Model file for the job. Use its own axes, mm. A direction names the side the tool comes from. Give positions to 0.01 mm unless a question says otherwise; leave off trailing zeros. Write each loop counter-clockwise with the first axis right and the second up, starting at its lowest first coordinate (ties: lowest second). Pieces come first, ordered by that corner, then holes. Notation, with made-up numbers: (15.5, 71.25) - (54.5, 71.25) arc R28 ccw to (54.5, 99.25) - close; hole circle Ø5 at (83.5, -12). An arc over 180 degrees is marked (long way). One line per item, written item: value. Start each with the question number.
(1) Drop flat-ended pins along their axis: P1, Ø1, axis at x = -4, z = 0, coming from the -Y side; P2, Ø4, axis at x = 0.5, y = 5.5, coming from the -Z side; P3, Ø0.9, axis at y = -1.5, z = -6.5, coming from the +X side; P4, Ø3, axis at x = 1.5, y = -1, coming from the +Z side. Give the stop position or say it passes through.
(2) Cut at A-A, the plane x = -4.75. List the corners of the cut face in (y, z), and give its area (3 significant figures).
(3) Cut at B-B, the plane y = 2.5. List the corners of the cut face in (x, z).
(4) Cut at D-D, the plane x = 0. List the corners of the cut face in (y, z).
(5) 3-axis set-ups, long thin cutter, end or side, ignore diameter. For faces 1 (the face through (-2.3, 3.1, -3.4)), 2 (the face through (-5.5, 1.5, -5.5)): which of +Z, -Z, +X, -X, +Y, -Y reach the whole face in a straight line?
(6) Cut at C-C, the plane z = 4. List the corners of the cut face in (x, y), and give its area (3 significant figures).
(7) Probe L1, parallel to Y at x = -2, z = 4.75; L2, parallel to Y at x = -5.5, z = 0.75; L3, parallel to Z at x = -2, y = 5. List the from-to ranges inside material, lowest first.
from build123d import *

# Parameters (mm, degrees)
SKETCH1_W            = 12
SKETCH1_H            = 12
BOSS_EXTRUDE1_DEPTH  = 3
CHAMFER1_SIZE        = 1
SKETCH2_W            = 10
SKETCH2_H            = 10
BOSS_EXTRUDE2_DEPTH  = 0.1
SKETCH3_R            = 0.5
BOSS_EXTRUDE3_DEPTH  = 0.05
LPATTERN1_COUNT      = 2
LPATTERN1_PITCH      = 8
LPATTERN1_COUNT_DIR2 = 2
LPATTERN1_PITCH_DIR2 = 8
SKETCH4_R            = 3.5
BOSS_EXTRUDE4_DEPTH  = 8
BOSS_EXTRUDE4_TAPER  = 4
SWEEP1_START         = -3
SWEEP1_DEPTH         = 1
SWEEP1_START_2       = 2
SWEEP1_2_DEPTH       = 1


# Read off the part's stored shape, not the designer's step: Dome1, Sweep1
with BuildPart() as part:
    # Sketch1 → Boss-Extrude1 (new body)
    with BuildSketch(Plane(origin=(0, 0, 0), x_dir=(1, 0, 0), z_dir=(0, 1, 0))):
        Rectangle(SKETCH1_W, SKETCH1_H)
    extrude(amount=BOSS_EXTRUDE1_DEPTH)

    # Chamfer1
    chamfer1_edges = [part.edges().sort_by_distance(p)[0] for p in [
        (6, 1.5, 6),
        (-6, 1.5, 6),
        (-6, 1.5, -6),
        (6, 1.5, -6),
    ]]
    chamfer(chamfer1_edges, length=CHAMFER1_SIZE)

    # Sketch2 → Boss-Extrude2 (add)
    with BuildSketch(Plane(origin=(0, 3, 0), x_dir=(1, 0, 0), z_dir=(0, 1, 0))):
        Rectangle(SKETCH2_W, SKETCH2_H)
    extrude(amount=BOSS_EXTRUDE2_DEPTH)

    # Sketch3 → Boss-Extrude3 (add)
    with BuildSketch(Plane(origin=(0, 3.1, 0), x_dir=(1, 0, 0), z_dir=(0, 1, 0))):
        with Locations(Location((-4, 4, 0), (0, 0, 270))):
            Circle(SKETCH3_R)
    boss_extrude3 = extrude(amount=BOSS_EXTRUDE3_DEPTH)

    # Dome1 outline → Dome1 (revolve)
    with BuildSketch(Plane(origin=(-4, 0, -4), x_dir=(1, 0, 0), z_dir=(0, 0, 1))):
        with BuildLine():
            Line((0, 3.15), (0.5, 3.149999999))
            ThreePointArc((0.5, 3.149999999), (0.353553391, 3.50355339), (0, 3.65))
            Line((0, 3.65), (0, 3.15))
        make_face()
    dome1 = revolve(axis=Axis((-4, 0, -4), (0, 1, 0)))

    # LPattern1: Boss-Extrude3, Dome1 2 × 2
    with Locations(*[(i * LPATTERN1_PITCH, 0, j * LPATTERN1_PITCH_DIR2) for i in range(LPATTERN1_COUNT) for j in range(LPATTERN1_COUNT_DIR2) if (i, j) != (0, 0)]):
        add(boss_extrude3)
        add(dome1)

    # Sketch4 → Boss-Extrude4 (add)
    with BuildSketch(Plane(origin=(0, 3.1, 0), x_dir=(1, 0, 0), z_dir=(0, 1, 0))):
        Circle(SKETCH4_R)
    extrude(amount=BOSS_EXTRUDE4_DEPTH, taper=BOSS_EXTRUDE4_TAPER)

    # Sweep1 outline → Sweep1 (add)
    with BuildSketch(Plane.YZ.offset(SWEEP1_START)):
        Polygon((0.75, 6), (-2.007966225, 6.818182656), (-4.321335721, 6.310463619), (-4.306093498, 6.241014001), (-2.010621634, 6.744805015), (0.5, 6), align=None)
    sweep1 = extrude(amount=SWEEP1_DEPTH)

    # Sweep1 2 outline → Sweep1 2 (add)
    with BuildSketch(Plane.YZ.offset(SWEEP1_START_2)):
        Polygon((0.75, 6), (-2.007966225, 6.818182656), (-4.321335721, 6.310463619), (-4.306093498, 6.241014001), (-2.010621634, 6.744805015), (0.5, 6), align=None)
    sweep1_2 = extrude(amount=SWEEP1_2_DEPTH)

    # Mirror1: Sweep1, Sweep1 2 across plane
    add(sweep1.mirror(Plane.XY))
    add(sweep1_2.mirror(Plane.XY))


solid = part.part
Answers follow:
1. P1: stops at y = 0
1. P2: stops at z = -3.47
1. P3: stops at x = 3
1. P4: stops at z = 6.82
2. outline: (0, -6) - (3, -6) - (3, -5) - (3.1, -5) - (3.1, 5) - (3, 5) - (3, 6) - (0, 6) - close
2. area: 37.0 mm²
3. outline: (-6, -5) - (-5, -6) - (5, -6) - (6, -5) - (6, 5) - (5, 6) - (-5, 6) - (-6, 5) - close
4. outline: (0, -6) - (3, -6) - (3, -5) - (3.1, -5) - (3.1, -3.5) - (11.1, -2.94) - (11.1, 2.94) - (3.1, 3.5) - (3.1, 5) - (3, 5) - (3, 6) - (0, 6) - close
5. face 1: +Y
5. face 2: -Z, -X, +Y, -Y
6. outline: (-6, 0) - (6, 0) - (6, 3) - (5, 3) - (5, 3.1) - (4.5, 3.1) - (4.5, 3.15) arc R0.5 ccw to (3.5, 3.15) - (3.5, 3.1) - (-3.5, 3.1) - (-3.5, 3.15) arc R0.5 ccw to (-4.5, 3.15) - (-4.5, 3.1) - (-5, 3.1) - (-5, 3) - (-6, 3) - close
6. area: 37.9 mm²
7. L1: y = 0 to 3.1
7. L2: y = 0 to 3
7. L3: z = -2.71 to 2.71
